Geometry: final body of the model. Coordinates: model frame, mm. Give positions to 0.01 mm unless a question says otherwise; leave off trailing zeros. Order: outer loops, then holes, each group sorted by start corner. A loop starts at its lowest first (then second) coordinate and runs counter-clockwise, first axis right, second up. Notation, with made-up numbers: (21.5, 32.5) -> (28.5, 32.5) arc R15 ccw to (28.5, 47.5) -> close; hole circle Ø3 at (71.5, 9). An arc over 180 degrees is marked (long way). One line per question, with ' | ' between items.
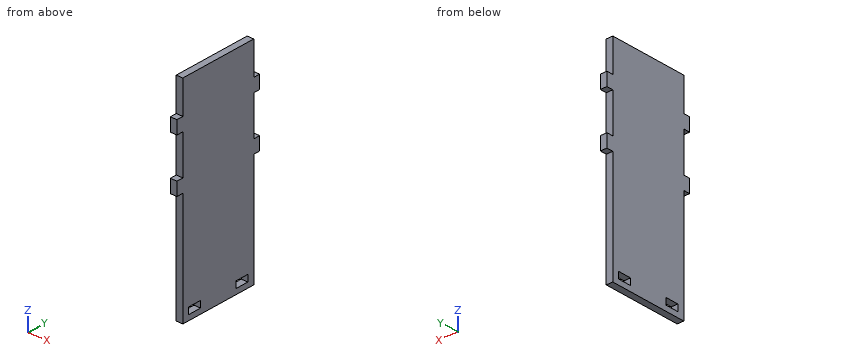
from build123d import *

# Parameters (mm, degrees)
SKETCH1_3_W         = 2.5
SKETCH1_3_H         = 5
SKETCH1_3_W_2       = 5
SKETCH1_3_H_2       = 2.5
SKETCH1_3_W_3       = 20
SKETCH1_3_H_3       = 30
BOSS_EXTRUDE2_DEPTH = 2.5


with BuildPart() as part:
    # Sketch1_3 → Boss-Extrude2 (new body)
    # profile 1 of 6: a face of its own
    with BuildSketch(Plane(origin=(0, 0, 0), x_dir=(0, 0, -1), z_dir=(1, 0, 0))):
        Polygon((-52.5, 15), (-57.5, 15), (-62.5, 15), (-67.5, 15), (-70, 15), (-70, -15), (-67.5, -15), (-62.5, -15), (-57.5, -15), (-52.5, -15), (-47.5, -15), (-42.5, -15), (-37.5, -15), (-32.5, -15), (-27.5, -15), (-22.5, -15), (-10, -15), (-10, 15), (-22.5, 15), (-27.5, 15), (-32.5, 15), (-37.5, 15), (-42.5, 15), (-47.5, 15), align=None)
        with Locations((-13.25, -10)):
            Rectangle(SKETCH1_3_W, SKETCH1_3_H, mode=Mode.SUBTRACT)
        with Locations((-13.25, 10)):
            Rectangle(SKETCH1_3_W, SKETCH1_3_H, mode=Mode.SUBTRACT)
    # profile 2 of 6: a face of its own
    with BuildSketch(Plane(origin=(0, 0, 0), x_dir=(0, 0, -1), z_dir=(1, 0, 0))):
        with Locations((-55, -16.25)):
            Rectangle(SKETCH1_3_W_2, SKETCH1_3_H_2)
    # profile 3 of 6: a face of its own
    with BuildSketch(Plane(origin=(0, 0, 0), x_dir=(0, 0, -1), z_dir=(1, 0, 0))):
        with Locations((-55, 16.25)):
            Rectangle(SKETCH1_3_W_2, SKETCH1_3_H_2)
    # profile 4 of 6: a face of its own
    with BuildSketch(Plane(origin=(0, 0, 0), x_dir=(0, 0, -1), z_dir=(1, 0, 0))):
        with Locations((-80, 0)):
            Rectangle(SKETCH1_3_W_3, SKETCH1_3_H_3)
    # profile 5 of 6: a face of its own
    with BuildSketch(Plane(origin=(0, 0, 0), x_dir=(0, 0, -1), z_dir=(1, 0, 0))):
        with Locations((-75, 16.25)):
            Rectangle(SKETCH1_3_W_2, SKETCH1_3_H_2)
    # profile 6 of 6: a face of its own
    with BuildSketch(Plane(origin=(0, 0, 0), x_dir=(0, 0, -1), z_dir=(1, 0, 0))):
        with Locations((-75, -16.25)):
            Rectangle(SKETCH1_3_W_2, SKETCH1_3_H_2)
    extrude(amount=BOSS_EXTRUDE2_DEPTH)


solid = part.part
1) Section C-C on z = 61. Return loops of the section in (x, y).
Check result:
outline: (0, -15) -> (2.5, -15) -> (2.5, 15) -> (0, 15) -> close
2) Section B-B on x = 0.65. Return loops of the section in (y, z).
Check result:
outline: (-17.5, 52.5) -> (-15, 52.5) -> (-15, 10) -> (15, 10) -> (15, 52.5) -> (17.5, 52.5) -> (17.5, 57.5) -> (15, 57.5) -> (15, 72.5) -> (17.5, 72.5) -> (17.5, 77.5) -> (15, 77.5) -> (15, 90) -> (-15, 90) -> (-15, 77.5) -> (-17.5, 77.5) -> (-17.5, 72.5) -> (-15, 72.5) -> (-15, 57.5) -> (-17.5, 57.5) -> close; hole (-12.5, 12) -> (-7.5, 12) -> (-7.5, 14.5) -> (-12.5, 14.5) -> close; hole (7.5, 12) -> (12.5, 12) -> (12.5, 14.5) -> (7.5, 14.5) -> close
3) Section A-A on y = -9. Return loops of the section in (x, z), plus the area to 3 significant figures.
Check result:
outline: (0, 10) -> (2.5, 10) -> (2.5, 12) -> (0, 12) -> close; (0, 14.5) -> (2.5, 14.5) -> (2.5, 90) -> (0, 90) -> close | area: 194 mm^2
4) Contact query for flat-ended pins moving along their axis: pin 1 Ø0.8 at (x, z) = (1.5, 13.5) entering from -Y; pin 2 Ø1.2 at (x, z) = (2, 41.5) entering from +Y. Output: stop coordinate, or through.
Check result:
pin 1: stops at y = -15 | pin 2: stops at y = 15
5) Material intervals for probe 1 along Y at (x, z) = (0.75, 14); probe 2 along Z at (x, y) = (1.85, -9.5); probe 3 along Z at (x, y) = (1.6, -16), sorted ascending. Write a range as from..to.
Check result:
probe 1: y = -15..-12.5, -7.5..7.5, 12.5..15 | probe 2: z = 10..12, 14.5..90 | probe 3: z = 52.5..57.5, 72.5..77.5
